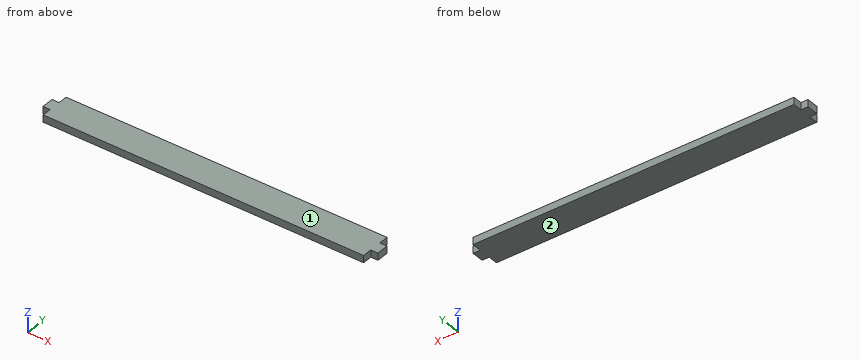
```python
from build123d import *

# Parameters (mm, degrees)
SKETCH1_W      = 5.9944
SKETCH1_H      = 10
EXTRUDE1_DEPTH = 5.9944


with BuildPart() as part:
    # Sketch1 → Extrude1 (new body)
    with BuildSketch(Plane.XY):
        Polygon((-209.134206709, 4.793644232), (58.827458806, 4.793644232), (58.827458806, 30.831866903), (-209.134206709, 30.234993462), align=None)
        with Locations((-212.131406709, 17.514318847)):
            Rectangle(SKETCH1_W, SKETCH1_H)
        with Locations((61.824658806, 17.812755567)):
            Rectangle(SKETCH1_W, SKETCH1_H)
    extrude(amount=EXTRUDE1_DEPTH)


solid = part.part
```
Geometry: final body of the model. Coordinates: model frame, mm. Face numbers are marked on the shaded views. Round coordinates to 2 decimals unless told otherwise and drop trailing zeros. Loops run counter-clockwise (first coordinate to the right, second up) from the corner with the lowest first, then second, coordinate; pieces in that order, holes last. Notation, with made-up numbers: (53.25, 5.5) -> (91.25, 5.5) arc R17 ccw to (91.25, 32.5) -> close; hole circle Ø10 at (3, 16.5). An arc over 180 degrees is marked (long way). Use one line per item in the form item = value. Start each with the question number.
1) Section C-C on x = -118. Output: boundary loops of the cut face in (y, z), then the cut area to 3 significant figures.
2) Line query: L1, parallel to X at y = 11.5, z = 1.65; L2, parallel to Y at x = 38.5, z = 4.45; L3, parallel to Y at x = 19, z = 3.85. Output: solid intervals per line, ascending.
3) Draft query along Z for the marked faces 1 and 2. Return one class per face: released by +Z, released by -Z, zero draft, split by the parting line, or undercut.
4) Section B-B on y = 27. Output: boundary loops of the cut face in (x, z), then the cut area to 3 significant figures.
5) Section A-A on z = 2. Output: boundary loops of the cut face in (x, y) (3 decimals), then the cut area to 3 significant figures.
6) First-contact query: P1, Ø1.8, axis at x = -212.5, z = 4, coming from the -Y side; P2, Ø3, axis at y = 28, z = 2.5, coming from the -X side; P3, Ø2, axis at x = -69, z = 1.5, coming from the +Y side. Flat tips, straight axial feed; report the tip coordinate or a pass-through.
Response:
q1.outline = (4.79, 0) -> (30.44, 0) -> (30.44, 5.99) -> (4.79, 5.99) -> close
q1.area = 154 mm^2
q2.L1 = -209.13 to 58.83
q2.L2 = 4.79 to 30.79
q2.L3 = 4.79 to 30.74
q3.face_1 = released by +Z
q3.face_2 = released by -Z
q4.outline = (-209.13, 0) -> (58.83, 0) -> (58.83, 5.99) -> (-209.13, 5.99) -> close
q4.area = 1,610 mm^2
q5.outline = (-215.129, 12.514) -> (-209.134, 12.514) -> (-209.134, 4.794) -> (58.827, 4.794) -> (58.827, 12.813) -> (64.822, 12.813) -> (64.822, 22.813) -> (58.827, 22.813) -> (58.827, 30.832) -> (-209.134, 30.235) -> (-209.134, 22.514) -> (-215.129, 22.514) -> close
q5.area = 7,020 mm^2
q6.P1 = 12.51
q6.P2 = -209.13
q6.P3 = 30.55
